Model file for the job. Use its own axes, mm. A direction names the side the tool comes from. Give positions to 0.01 mm unless a question says otherwise; leave off trailing zeros. Write each loop counter-clockwise with the first axis right and the second up, starting at its lowest first coordinate (ties: lowest second). Pieces come first, ordered by that corner, then holes.
```python
from build123d import *

# Parameters (mm, degrees)
SKETCH1_R             = 1.143
BOSS_EXTRUDE1_DEPTH   = 1.524
BOSS_EXTRUDE1_2_DEPTH = 1.524
SKETCH2_R             = 1.143
CUT_EXTRUDE2_DEPTH    = 26.441049651
SKETCH3_R             = 1.143
BOSS_EXTRUDE2_DEPTH   = 3.048


with BuildPart() as part:
    # Sketch1 → Boss-Extrude1 (new, symmetric)
    with BuildSketch(Plane(origin=(0, 0, 0), x_dir=(1, 0, 0), z_dir=(0, 1, 0))):
        with BuildLine():
            Line((-14.395123673, -5.0038), (-16.984058744, -5.5245))
            ThreePointArc((-16.984058744, -5.5245), (10.284594762, -14.601556843), (10.922, 14.131109924))
            Line((10.922, 14.131109924), (10.922, 10.9728))
            Line((10.922, 10.9728), (11.43, 10.9728))
            Line((11.43, 10.9728), (11.43, -0.8128))
            Line((11.43, -0.8128), (12.9413, -0.8128))
            Line((12.9413, -0.8128), (12.9413, -4.064))
            Line((12.9413, -4.064), (8.4582, -4.064))
            Line((8.4582, -4.064), (8.4582, -8.9154))
            Line((8.4582, -8.9154), (1.2573, -8.9154))
            Line((1.2573, -8.9154), (1.2573, -7.3406))
            Line((1.2573, -7.3406), (-0.7747, -8.8265))
            Line((-0.7747, -8.8265), (-3.273729572, -11.3919))
            Line((-3.273729572, -11.3919), (-5.093162196, -9.619538602))
            Line((-5.093162196, -9.619538602), (-4.769706241, -9.287492148))
            Line((-4.769706241, -9.287492148), (-9.167166743, -5.0038))
            Line((-9.167166743, -5.0038), (-14.395123673, -5.0038))
        make_face()
        with Locations(Location((0, -13.2588, 0), (0, 0, 90))):
            Circle(SKETCH1_R, mode=Mode.SUBTRACT)
        with Locations(Location((10.832526773, -7.6454, 0), (0, 0, 90))):
            Circle(SKETCH1_R, mode=Mode.SUBTRACT)
    extrude(amount=BOSS_EXTRUDE1_DEPTH, both=True)


with BuildPart() as body_2:
    # Sketch1 → Boss-Extrude1 2 (new, symmetric)
    with BuildSketch(Plane(origin=(0, 0, 0), x_dir=(1, 0, 0), z_dir=(0, 1, 0))):
        with BuildLine():
            Line((-4.179129857, 14.6558), (10.207148379, 14.6558))
            ThreePointArc((10.207148379, 14.6558), (-5.685665172, 16.930787437), (-16.984058744, 5.5245))
            Line((-16.984058744, 5.5245), (-14.203432675, 5.5245))
            ThreePointArc((-14.203432675, 5.5245), (-13.378320264, 7.299188099), (-12.332576282, 8.9535))
            Line((-12.332576282, 8.9535), (-7.9248, 7.366))
            Line((-7.9248, 7.366), (-7.9248, 3.302))
            Line((-7.9248, 3.302), (-5.6007, 3.302))
            Line((-5.6007, 3.302), (-5.6007, 14.173558463))
            ThreePointArc((-5.6007, 14.173558463), (-4.895856129, 14.43219293), (-4.179129857, 14.6558))
        make_face()
        with Locations(Location((-8.579035657, 10.1092, 0), (0, 0, 90))):
            Circle(SKETCH1_R, mode=Mode.SUBTRACT)
    extrude(amount=BOSS_EXTRUDE1_2_DEPTH, both=True)


with BuildPart() as cut_extrude2_tool:
    # Sketch2 → Cut-Extrude2 (new, through all)
    # profile 1 of 3: a face of its own
    with BuildSketch(Plane(origin=(0, 1.524, 0), x_dir=(1, 0, 0), z_dir=(0, 1, 0))):
        with BuildLine():
            Line((-12.676023011, 12.581605315), (-9.741012668, 9.123103947))
            ThreePointArc((-9.741012668, 9.123103947), (-7.592939604, 8.947222989), (-7.417058645, 11.095296053))
            Line((-7.417058645, 11.095296053), (-10.352068988, 14.55379742))
            ThreePointArc((-10.352068988, 14.55379742), (-11.556194906, 13.61736799), (-12.676023011, 12.581605315))
        make_face()
        with Locations((-8.579035657, 10.1092)):
            Circle(SKETCH2_R, mode=Mode.SUBTRACT)
    # profile 2 of 3: a face of its own
    with BuildSketch(Plane(origin=(0, 1.524, 0), x_dir=(1, 0, 0), z_dir=(0, 1, 0))):
        with BuildLine():
            Line((1.524, -17.794824407), (1.524, -13.2588))
            ThreePointArc((1.524, -13.2588), (0, -11.7348), (-1.524, -13.2588))
            Line((-1.524, -13.2588), (-1.524, -17.794824407))
            ThreePointArc((-1.524, -17.794824407), (0, -17.859965052), (1.524, -17.794824407))
        make_face()
        with Locations((0, -13.2588)):
            Circle(SKETCH2_R, mode=Mode.SUBTRACT)
    # profile 3 of 3: a face of its own
    with BuildSketch(Plane(origin=(0, 1.524, 0), x_dir=(1, 0, 0), z_dir=(0, 1, 0))):
        with BuildLine():
            Line((9.953745163, -8.89051802), (13.659706927, -11.506118301))
            ThreePointArc((13.659706927, -11.506118301), (14.591708872, -10.298562224), (15.417270145, -9.015882261))
            Line((15.417270145, -9.015882261), (11.711308382, -6.40028198))
            ThreePointArc((11.711308382, -6.40028198), (9.587408753, -6.766618391), (9.953745163, -8.89051802))
        make_face()
        with Locations((10.832526773, -7.6454)):
            Circle(SKETCH2_R, mode=Mode.SUBTRACT)
    extrude(amount=-CUT_EXTRUDE2_DEPTH)


with BuildPart() as part_1:
    add(part.part)

    # Cut-Extrude2: cut by cut_extrude2_tool
    add(cut_extrude2_tool.part, mode=Mode.SUBTRACT)



with BuildPart() as body_2_1:
    add(body_2.part)

    # Cut-Extrude2: cut by cut_extrude2_tool
    add(cut_extrude2_tool.part, mode=Mode.SUBTRACT)


with BuildPart() as part_2:
    add(part_1.part)

    add(body_2_1.part)  # Boss-Extrude2 merges body 2
    # Sketch3 → Boss-Extrude2 (add)
    # profile 1 of 2: a face of its own
    with BuildSketch(Plane(origin=(0, 1.524, 0), x_dir=(1, 0, 0), z_dir=(0, 1, 0))):
        with BuildLine():
            ThreePointArc((6.893924032, 16.475805386), (8.598824007, 15.653708103), (10.207148379, 14.6558))
            Line((10.207148379, 14.6558), (10.922, 14.6558))
            Line((10.922, 14.6558), (10.922, 14.131109924))
            ThreePointArc((10.922, 14.131109924), (12.114466388, 13.123187715), (13.214344503, 12.014967792))
            ThreePointArc((13.214344503, 12.014967792), (12.840241174, 13.300024042), (13.624339722, 14.384695574))
            ThreePointArc((13.624339722, 14.384695574), (13.960152262, 19.779700621), (8.989376751, 17.655967979))
            ThreePointArc((8.989376751, 17.655967979), (8.230051983, 16.553811563), (6.893924032, 16.475805386))
        make_face()
        with Locations(Location((12.129357243, 17.185704746, 0), (0, 0, 270))):
            Circle(SKETCH3_R, mode=Mode.SUBTRACT)
    # profile 2 of 2: a face of its own
    with BuildSketch(Plane(origin=(0, 1.524, 0), x_dir=(1, 0, 0), z_dir=(0, 1, 0))):
        with BuildLine():
            ThreePointArc((-13.214344503, -12.014967792), (-12.840241174, -13.300024042), (-13.624339722, -14.384695574))
            ThreePointArc((-13.624339722, -14.384695574), (-13.960152262, -19.779700621), (-8.989376751, -17.655967979))
            ThreePointArc((-8.989376751, -17.655967979), (-8.230051983, -16.553811563), (-6.893924032, -16.475805386))
            ThreePointArc((-6.893924032, -16.475805386), (-10.298562224, -14.591708872), (-13.214344503, -12.014967792))
        make_face()
        with Locations(Location((-12.129357243, -17.185704746, 0), (0, 0, 270))):
            Circle(SKETCH3_R, mode=Mode.SUBTRACT)
    extrude(amount=-BOSS_EXTRUDE2_DEPTH)


solid = part_2.part
```
1. Pin check, flat tips, straight feed: P1, Ø2, axis at x = -12.13, z = 17.19, coming from the +Y side; P2, Ø1.5, axis at x = -12, y = 0.5, coming from the -Z side; P3, Ø0.8, axis at x = 12, y = -0.5, coming from the +Z side; P4, Ø1.7, axis at y = 0.5, z = 8, coming from the +X side. Stop position of each tip, or through.
Calculated:
P1: passes through
P2: stops at z = -12.58
P3: stops at z = 13.58
P4: stops at x = 16.37
2. Probe probe 1 along Z at (x, y) = (10, 0.55); probe 2 along Z at (x, y) = (-12.5, 0); probe 3 along Z at (x, y) = (-5.5, -1). List the from-to ranges inside material, lowest first.
Calculated:
probe 1: z = -19.54 to -14.66, 4.06 to 6.37, 8.92 to 14.8
probe 2: z = -12.37 to -8.72, 5 to 16.1, 18.27 to 20.34
probe 3: z = -16.99 to -14.21, 8.58 to 16.99
3. Slice it at A-A, the plane x = 0. Write the cut outline in (y, z), and give its area (3 significant figures).
Calculated:
outline: (-1.52, -17.86) - (1.52, -17.86) - (1.52, -14.66) - (-1.52, -14.66) - close; (-1.52, 8.26) - (1.52, 8.26) - (1.52, 11.73) - (-1.52, 11.73) - close
area: 20.4 mm2
4. Which spindle directions (+Z, -Z, +X, -X, +Y, -Y) get a long thin tool onto all of the face, cutting with end or side? Do faces 1 (the cylindrical face through (-15.21, 0.02, -9.36)), 2 (the flat face through (4, 1.524, 10)), 3 (the cylindrical face through (-15.471, 0.021, 8.924)), 4 (the flat face through (0.26, 0.02, 8.07)), 5 (the cylindrical face through (-4.298, 0.021, 17.335)). Say none if no direction does.
Calculated:
face 1: -Z, -X, +Y, -Y
face 2: +Z, -Z, +X, -X, +Y
face 3: -X, +Y, -Y
face 4: +Y, -Y
face 5: +Z, +Y, -Y
5. Slice it at C-C, the plane x = 4. Write the cut outline in (y, z).
Calculated:
outline: (-1.52, -17.41) - (1.52, -17.41) - (1.52, -14.66) - (-1.52, -14.66) - close; (-1.52, 8.92) - (1.52, 8.92) - (1.52, 17.41) - (-1.52, 17.41) - close
6. Slice it at D-D, the plane z = -1.5. Write the cut outline in (x, y).
Calculated:
outline: (11.43, -1.52) - (17.8, -1.52) - (17.8, 1.52) - (11.43, 1.52) - close
7. Slice it at B-B, the plane y = -0.5. State how many separate pieces and enclosed holes the cut face has, and give its area (3 significant figures).
Calculated:
separate pieces: 1
enclosed holes: 2
area: 474 mm2
